Build history of the part. All positions in model axes, mm. Face numbers are marked on the shaded views. A direction names the side the tool comes from. Round coordinates to 2 decimals unless told otherwise and drop trailing zeros. Write each loop counter-clockwise with the first axis right and the second up, starting at its lowest first coordinate (ties: lowest second). Pieces come first, ordered by that corner, then holes. Notation, with made-up numbers: (74.25, 49.25) -> (107.25, 49.25) arc R15 cw to (107.25, 66.25) -> close; hole circle Ø2 at (78.5, 61.5). An arc over 180 degrees is marked (long way). Answer in a Markdown table with one row per item.
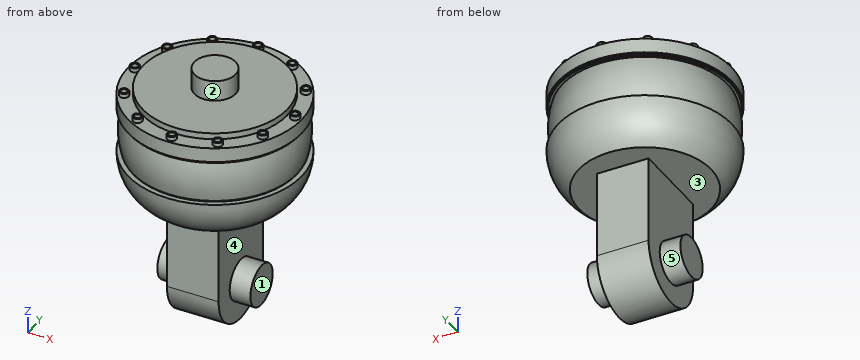
```python
from build123d import *

# Parameters (mm, degrees)
SKETCH2_R           = 39.5
BOSS_EXTRUDE1_DEPTH = 1
SKETCH4_R           = 41.25
BOSS_EXTRUDE2_DEPTH = 1
SKETCH5_R           = 42
BOSS_EXTRUDE3_DEPTH = 7
SKETCH6_R           = 35
BOSS_EXTRUDE4_DEPTH = 3
SKETCH7_R           = 2.25
SKETCH7_R_2         = 1.5
BOSS_EXTRUDE5_DEPTH = 2
CIRPATTERN1_COUNT   = 12
SKETCH8_W           = 25
SKETCH8_H           = 40
BOSS_EXTRUDE6_DEPTH = 42
SKETCH9_R           = 20
BOSS_EXTRUDE7_DEPTH = 25
SKETCH10_R          = 10
BOSS_EXTRUDE8_DEPTH = 10
SKETCH11_R          = 10
BOSS_EXTRUDE9_DEPTH = 10


with BuildPart() as part:
    # Sketch1 → Revolve1 (revolve)
    with BuildSketch(Plane(origin=(0, 0, 0), x_dir=(1, 0, 0), z_dir=(0, 1, 0)), mode=Mode.PRIVATE) as revolve1_sk:
        with BuildLine():
            Line((-42, 0), (0, 0))
            Line((0, 0), (0, 20))
            Line((0, 20), (-32, 20))
            ThreePointArc((-32, 20), (-39.360679775, 11.180339887), (-42, 0))
        make_face()
    revolve(revolve1_sk.sketch.rotate(Axis((0, 0, 0), (0, 0, -1)), 180), axis=Axis((0, 0, 0), (0, 0, -1)))

    # Sketch2 → Boss-Extrude1 (add)
    with BuildSketch(Plane.XY):
        Circle(SKETCH2_R)
    extrude(amount=BOSS_EXTRUDE1_DEPTH)

    # Sketch3 → Revolve2 (revolve)
    with BuildSketch(Plane(origin=(0, 0, 0), x_dir=(1, 0, 0), z_dir=(0, 1, 0)), mode=Mode.PRIVATE) as revolve2_sk:
        with BuildLine():
            Line((0, -1), (0, -21))
            Line((0, -21), (-40, -21))
            ThreePointArc((-40, -21), (-41.376973739, -11), (-40, -1))
            Line((-40, -1), (0, -1))
        make_face()
    revolve(revolve2_sk.sketch.rotate(Axis((0, 0, 1), (0, 0, 1)), 180), axis=Axis((0, 0, 1), (0, 0, 1)))

    # Sketch4 → Boss-Extrude2 (add)
    with BuildSketch(Plane.XY.offset(21)):
        Circle(SKETCH4_R)
    extrude(amount=BOSS_EXTRUDE2_DEPTH)

    # Sketch5 → Boss-Extrude3 (add)
    with BuildSketch(Plane.XY.offset(22)):
        Circle(SKETCH5_R)
    extrude(amount=BOSS_EXTRUDE3_DEPTH)

    # Sketch6 → Boss-Extrude4 (add)
    with BuildSketch(Plane.XY.offset(29)):
        Circle(SKETCH6_R)
    extrude(amount=BOSS_EXTRUDE4_DEPTH)

    # Sketch7 → Boss-Extrude5 (add)
    with BuildSketch(Plane.XY.offset(29)):
        with Locations((38.75, 0)):
            Circle(SKETCH7_R)
        with Locations((38.75, 0)):
            Circle(SKETCH7_R_2, mode=Mode.SUBTRACT)
    boss_extrude5 = extrude(amount=BOSS_EXTRUDE5_DEPTH)

    # CirPattern1: Boss-Extrude5 ×12 about axis
    cirpattern1_axis = Axis((0, 0, 0), (0, 0, 1))
    for i in range(1, CIRPATTERN1_COUNT):
        add(boss_extrude5.rotate(cirpattern1_axis, i * 360 / CIRPATTERN1_COUNT))

    # Sketch8 → Boss-Extrude6 (add)
    with BuildSketch(Plane(origin=(0, 0, -20), x_dir=(-1, 0, 0), z_dir=(0, 0, -1))):
        Rectangle(SKETCH8_W, SKETCH8_H)
    extrude(amount=BOSS_EXTRUDE6_DEPTH)

    # Sketch9 → Boss-Extrude7 (add)
    with BuildSketch(Plane.ZY.offset(12.5)):
        with Locations((-62, 0)):
            Circle(SKETCH9_R)
    extrude(amount=-BOSS_EXTRUDE7_DEPTH)

    # Sketch10 → Boss-Extrude8 (add)
    with BuildSketch(Plane.ZY.offset(12.5)):
        with Locations(Location((-62, 0, 0), (0, 0, 90))):
            Circle(SKETCH10_R)
    boss_extrude8 = extrude(amount=BOSS_EXTRUDE8_DEPTH)

    # Mirror1: Boss-Extrude8 across plane
    add(boss_extrude8.mirror(Plane(origin=(0, 0, 0), x_dir=(0, 0, 1), z_dir=(1, 0, 0))))

    # Sketch11 → Boss-Extrude9 (add)
    with BuildSketch(Plane.XY.offset(32)):
        Circle(SKETCH11_R)
    extrude(amount=BOSS_EXTRUDE9_DEPTH)


solid = part.part
```
Q1. Wall check: line 1 (Y direction, x = 38.75, z = 30.35); line 2 (X direction, y = 18.5, z = -61); line 3 (Z direction, x = 20, y = 13.5). Give the ranges that are in metal, low to high. Write a range as [from, to].
A:
| item | result |
|---|---|
| line 1 | [-2.25, -1.5], [1.5, 2.25] |
| line 2 | [-12.5, 12.5] |
| line 3 | [-20, 32] |
Q2. Which spindle directions (+Z, -Z, +X, -X, +Y, -Y) get a long thin tool onto all of the face, cutting with end or side? Do the marked faces 1, 2, 3, 4 and 5. Say none if no direction does.
A:
| item | result |
|---|---|
| face 1 | -Z, +X, +Y, -Y |
| face 2 | +Z |
| face 3 | none |
| face 4 | +X |
| face 5 | -X |
Q3. Drop flat-ended pins along their axis: P1, Ø0.9, axis at x = -20, y = -33.5, coming from the +Z side; P2, Ø1.5, axis at x = 23.5, z = 22, coming from the -Y side; P3, Ø8, axis at x = -12.5, z = -51.5, coming from the +Y side; P4, Ø25, axis at x = 15, y = 15.5, coming from the +Z side. Give the stop position or say it passes through.
A:
| item | result |
|---|---|
| P1 | z = 29 |
| P2 | y = -35.3 |
| P3 | y = 20 |
| P4 | z = 42 |
Q4. Saw through at A-A on z = -59. Write the cut outline in (x, y), plus the area to 3 significant figures.
A:
| item | result |
|---|---|
| outline | (-22.5, -9.54) -> (-12.5, -9.54) -> (-12.5, -20) -> (12.5, -20) -> (12.5, -9.54) -> (22.5, -9.54) -> (22.5, 9.54) -> (12.5, 9.54) -> (12.5, 20) -> (-12.5, 20) -> (-12.5, 9.54) -> (-22.5, 9.54) -> close |
| area | 1,380 mm² |
